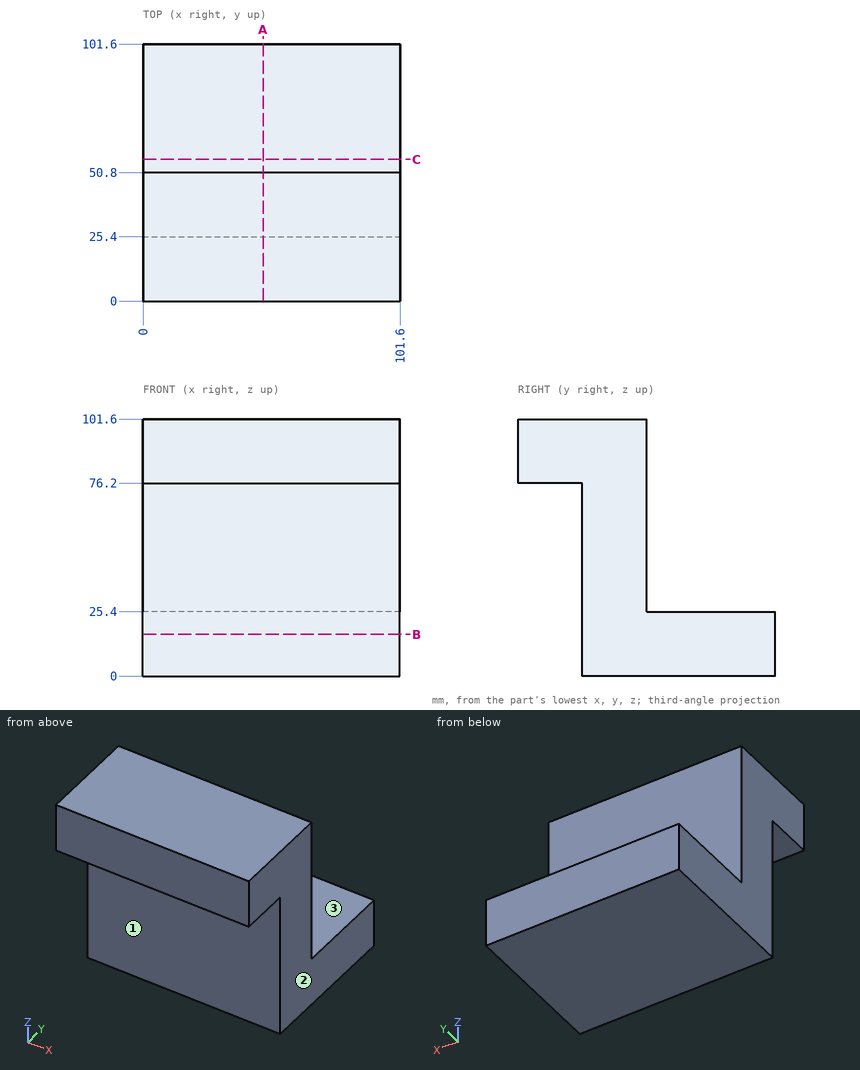
Answer from the drawing. Dimensions are ordinates in mm from the lowest x, y and z of the part. A direction names the side the tool comes from. Round coordinates to 2 decimals unless told otherwise and drop trailing zeros. Order: outer loops, then holes, each group sorted by start corner. A loop starts at its lowest first (then second) coordinate and runs counter-clockwise, first axis right, second up. Notation, with made-up numbers: (-1.75, 21) -> (31.25, 21) arc R29 ccw to (31.25, 45) -> close; hole circle Ø8 at (30, 15.5). An arc over 180 degrees is marked (long way). Answer as CSV lines item,"result".
Q1. A cutting plane is placed at A-A on x = 47.5. Determine the outline of the cut face in (y, z), plus the area to 3 significant figures.
Computed values:
outline,"(0, 76.2) -> (25.4, 76.2) -> (25.4, 0) -> (101.6, 0) -> (101.6, 25.4) -> (50.8, 25.4) -> (50.8, 101.6) -> (0, 101.6) -> close"
area,"4,520 mm^2"
Q2. Given pin 1 (6 mm diameter, centred on x = 11.5, z = 13.5, fed in from -Y); pin 2 (6 mm diameter, centred on y = 91.5, z = 29, fed in from -X); pin 3 (12.5 mm diameter, centred on x = 33.5, y = 18.5, fed in from -Z); pin 4 (2 mm diameter, centred on x = 39, z = 25.5, fed in from +Y), each flat-ended and moving along its own axis, determine where each tip first touches the part or whether it passes through.
Computed values:
pin 1,"stops at y = 25.4"
pin 2,"passes through"
pin 3,"stops at z = 76.2"
pin 4,"stops at y = 101.6"
Q3. A cutting plane is placed at C-C on y = 56. Determine the outline of the cut face in (x, z).
Computed values:
outline,"(0, 0) -> (101.6, 0) -> (101.6, 25.4) -> (0, 25.4) -> close"
Q4. A cutting plane is placed at B-B on z = 16.5. Determine the outline of the cut face in (x, y).
Computed values:
outline,"(0, 25.4) -> (101.6, 25.4) -> (101.6, 101.6) -> (0, 101.6) -> close"
Q5. Consider line 1 (Y direction, x = 64.5, z = 29.5); line 2 (Z direction, x = 61, y = 93.5); line 3 (Z direction, x = 76, y = 7.5). Determine where each line is inside the solid, lowest interval first. Write a range as from..to.
Computed values:
line 1,"y = 25.4..50.8"
line 2,"z = 0..25.4"
line 3,"z = 76.2..101.6"
Q6. Which of the six approach directions +Z, -Z, +X, -X, +Y, -Y give full straight-line access (tool end or side, diameter ignored) to the marked faces 1, 2 and 3?
Computed values:
face 1,"-Z, +X, -X, -Y"
face 2,"+Z, -Z, +X, +Y, -Y"
face 3,"+Z, +X, -X, +Y"
